Here's how the part is built. I have some questions about the finished solid (model axes, mm). Give positions to 0.01 mm unless a question says otherwise; leave off trailing zeros. Loops run counter-clockwise (first coordinate to the right, second up) from the corner with the lowest first, then second, coordinate; pieces in that order, holes last.
Q1. If we section it at B-B (y = -193): Please give me the cut outline in (x, z) (3 decimals).
Q2. I need wall thicknesses on line 1 (Y direction, x = 3, z = 297); line 2 (Y direction, x = 8.5, z = 40); line 3 (Z direction, x = 1.5, y = -163). Which ranges of each line are inside material? Lowest first, please.
Q3. If we section it at C-C (z = 277.5): Please give me the cut outline in (x, y) (3 decimals).
Q4. If we section it at A-A (x = 2): Give the number of separate pieces and of enclosed holes in the cut face, plus the area to 3 significant figures.
Q5. Will these pins go through, and if not, where does the flat tip stop? P1, Ø5, axis at x = 3.5, z = 312, coming from the -Y side; P2, Ø1.5, axis at x = 1.5, y = -286, coming from the -Z side; P3, Ø3, axis at x = 5, y = -271, coming from the +Z side.
from build123d import *

# Parameters (mm, degrees)
F0_W     = 127
F0_H     = 406.4
F1_DEPTH = 9.525
F3_DEPTH = 9.525
F4_R     = 63.49999
F6_D     = 20.6375
F8_D     = 20.6375


# Not quite as in the source:
# - a fillet or chamfer is up to 0.001 mm smaller than in the source, because OpenCascade refuses the exact size
# - a length typed as a fraction of an inch, garbled in the dataset ("3 / 203.2 mm" for 3/8 in), is restored


with BuildPart() as f1:
    # F0 (on Right) → F1 (new body)
    with BuildSketch(Plane.YZ):
        with Locations((26.2075642347, 169.2136289895)):
            Rectangle(F0_W, F0_H)
    extrude(amount=F1_DEPTH)

    # F2 (on face) → F3 (join)
    with BuildSketch(Plane.YZ.offset(9.525)):
        Polygon((-37.2924357653, 105.7136289895), (-37.2924357653, 169.2136289895), (-37.2924357653, 232.7136289895), (-354.7924357653, 232.7136289895), (-354.7924357653, 105.7136289895), align=None)
    extrude(amount=-F3_DEPTH)

    # F4 (radius 63.5 in the source; OpenCascade refuses exactly that, so slightly less here)
    f4_edges = [f1.edges().sort_by_distance(p)[0] for p in [
        (4.7625, -354.792436, 232.713629),
        (4.7625, -354.792436, 105.713629),
    ]]
    fillet(f4_edges, radius=F4_R)

    # F6 (through all)
    with Locations(Plane.YZ.offset(9.525)):
        with Locations((-291.2924357653, 169.2136289895)):
            Hole(F6_D / 2)

    # F8 (through all)
    with Locations(Plane.YZ.offset(9.525)):
        with Locations((26.2075642347, 296.2136289895), (26.2075642347, 194.6136289895), (26.2075642347, 93.0136289895), (26.2075642347, -8.5863710105)):
            Hole(F8_D / 2)


solid = f1.part
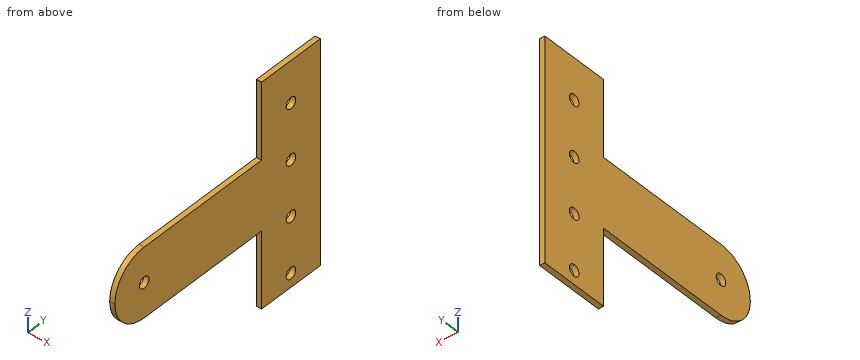
Check sheet entries:
1. outline: (0, 105.714) - (9.525, 105.714) - (9.525, 232.714) - (0, 232.714) - close
2. line 1: y = -37.29 to 15.92, 36.5 to 89.71
2. line 2: y = -37.29 to 89.71
2. line 3: z = 105.71 to 232.71
3. outline: (0, -37.292) - (9.525, -37.292) - (9.525, 89.708) - (0, 89.708) - close
4. separate pieces: 1
4. enclosed holes: 5
4. area: 88,500 mm2
5. P1: stops at y = -37.29
5. P2: stops at z = 105.71
5. P3: stops at z = 232.71
